Geometry check sheet. Reference: the model listing, model coordinates, mm. Give positions to 0.01 mm unless a question says otherwise; leave off trailing zeros. Loops run counter-clockwise (first coordinate to the right, second up) from the corner with the lowest first, then second, coordinate; pieces in that order, holes last. Notation, with made-up numbers: (35, 16.5) -> (91, 16.5) arc R19 ccw to (91, 35.5) -> close; hole circle Ø10 at (64.5, -26). An arc over 180 degrees is marked (long way). Write item = value, one per line. Start each with the question number.
```python
from build123d import *

# Parameters (mm, degrees)
ESQUISSE1_W                                 = 100
ESQUISSE1_H                                 = 100
BOSS_EXTRU_1_DEPTH                          = 3
FRAISAGE_POUR_VIS_T_TE_FRAIS_E_M31_AT_COUNT = 2
FRAISAGE_POUR_VIS_T_TE_FRAIS_E_M31_AT_PITCH = 90
FRAISAGE_POUR_VIS_T_TE_FRAIS_E_M31_2_COUNT  = 2
FRAISAGE_POUR_VIS_T_TE_FRAIS_E_M31_2_PITCH  = 127.279220614
FRAISAGE_POUR_VIS_T_TE_FRAIS_E_M31_3_COUNT  = 2
FRAISAGE_POUR_VIS_T_TE_FRAIS_E_M31_3_PITCH  = 90


with BuildPart() as part:
    # Esquisse1 → Boss.-Extru.1 (new body)
    with BuildSketch(Plane.XY):
        with Locations((50, 50)):
            Rectangle(ESQUISSE1_W, ESQUISSE1_H)
    extrude(amount=BOSS_EXTRU_1_DEPTH)

    # Esquisse3 → Fraisage pour vis à tête fraisée M31 (revolve, cut)
    with BuildSketch(Plane(origin=(5, 95, 3), x_dir=(0, -1, 0), z_dir=(1, 0, 0))):
        Polygon((0, 0), (0, 3), (1.8, 3), (1.8, 1.35), (3.15, 0), align=None)
    fraisage_pour_vis_t_te_frais_e_m31 = revolve(axis=Axis((5, 95, 9.35), (0, 0, -1)), mode=Mode.SUBTRACT)

    # Fraisage pour vis à tête fraisée M31 at: Fraisage pour vis à tête fraisée M31 ×2
    with Locations(*[(i * FRAISAGE_POUR_VIS_T_TE_FRAIS_E_M31_AT_PITCH, 0, 0) for i in range(1, FRAISAGE_POUR_VIS_T_TE_FRAIS_E_M31_AT_COUNT)]):
        add(fraisage_pour_vis_t_te_frais_e_m31, mode=Mode.SUBTRACT)

    # Fraisage pour vis _ t_te frais_e M31 2: Fraisage pour vis à tête fraisée M31 ×2
    with Locations(*[Vector(0.707106781, -0.707106781, 0) * (i * FRAISAGE_POUR_VIS_T_TE_FRAIS_E_M31_2_PITCH) for i in range(1, FRAISAGE_POUR_VIS_T_TE_FRAIS_E_M31_2_COUNT)]):
        add(fraisage_pour_vis_t_te_frais_e_m31, mode=Mode.SUBTRACT)

    # Fraisage pour vis _ t_te frais_e M31 3: Fraisage pour vis à tête fraisée M31 ×2
    with Locations(*[(0, -i * FRAISAGE_POUR_VIS_T_TE_FRAIS_E_M31_3_PITCH, 0) for i in range(1, FRAISAGE_POUR_VIS_T_TE_FRAIS_E_M31_3_COUNT)]):
        add(fraisage_pour_vis_t_te_frais_e_m31, mode=Mode.SUBTRACT)


solid = part.part
```
1) Thickness scan on line 1 (X direction, y = 95, z = 0.95). Record the ranges inside material, lowest first.
2) Draft check along Y on faces 1 (the flat face through (49, 0, 1)), 2 (the cylindrical face through (5.689, 3.337, 0.837)), 3 (the flat face through (100, 49, 1)). Enter one of: released by +Y, released by -Y, zero draft, split by the parting line, or undercut.
3) Depth check by flat-ended pin: pin 1 Ø3 at (x, y) = (5, 5) entering from -Z; pin 2 Ø4 at (x, y) = (95, 5) entering from +Z. Enter the tip coordinate at first touch or a pass-through.
4) Section check A-A (x = 5). Enter the section's corners in (y, z), plus the area to 3 significant figures.
Check result:
q1.line_1 = 0 to 3.2, 6.8 to 93.2, 96.8 to 100
q2.face_1 = released by -Y
q2.face_2 = undercut
q2.face_3 = zero draft
q3.pin_1 = through
q3.pin_2 = 1.85
q4.outline = (0, 0) -> (3.2, 0) -> (3.2, 1.65) -> (1.85, 3) -> (0, 3) -> close; (6.8, 0) -> (93.2, 0) -> (93.2, 1.65) -> (91.85, 3) -> (8.15, 3) -> (6.8, 1.65) -> close; (96.8, 0) -> (100, 0) -> (100, 3) -> (98.15, 3) -> (96.8, 1.65) -> close
q4.area = 275 mm2
